CAD build for the part. Positions are in the model's coordinates, mm. Face numbers are marked on the shaded views. A direction names the side the tool comes from. Give positions to 0.01 mm unless a question says otherwise; leave off trailing zeros. Write each loop counter-clockwise with the first axis right and the second up, starting at its lowest first coordinate (ties: lowest second). Pieces come first, ordered by that corner, then holes. Notation, with made-up numbers: M -12,-25 L 22,-25 A30 ccw 22,14 Z; hole C 54.25,79.5 d7. An arc over 180 degrees is marked long. One line per question, with ' | ' between items. Start each with the question number.
1. Cut at A-A, the plane z = 0. Write the cut outline in (x, y).
2. Cut at B-B, the plane y = 10.5. Write the cut outline in (x, z).
3. Cut at D-D, the plane y = 5.75. Write the cut outline in (x, z), then the cut area to 3 significant figures.
4. Which spindle directions (+Z, -Z, +X, -X, +Y, -Y) get a long thin tool onto all of the face, cutting with end or side? Do the marked faces 1 and 2. Say none if no direction does.
5. Flat gauge pins, fed straight in: pin 1 (8 mm diameter, centred on x = 29.5, z = 37.5, fed in from +Y); pin 2 (5 mm diameter, centred on x = 10.5, y = 6, fed in from -Z); pin 3 (0.6 mm diameter, centred on y = 3, z = 0, fed in from +X); pin 4 (3.5 mm diameter, centred on x = 0, z = 0, fed in from +Y). Where does each tip first touch, or does it go through?
6. Wall check: L1, parallel to X at y = 3.2, z = 0; L2, parallel to X at y = 1.5, z = 0; L3, parallel to Z at x = -1, y = 3. Give the ranges that are in metal, low to high.
7. Cut at C-C, the plane x = 0. Write the cut outline in (y, z), then the cut area to 3 significant figures.
```python
from build123d import *

# Parameters (mm, degrees)
BOSS_EXTRUDE1_DEPTH = 9
SKETCH2_W           = 4
SKETCH2_H           = 20
BOSS_EXTRUDE2_DEPTH = 17
SKETCH3_W           = 15
SKETCH3_H           = 5
CUT_EXTRUDE1_DEPTH  = 66.094162565
SKETCH4_R           = 3
CUT_EXTRUDE2_DEPTH  = 68.830671528
CUT_EXTRUDE3_DEPTH  = 73.919476136
CUT_EXTRUDE4_DEPTH  = 71.606302835
FILLET1_R           = 5
CHAMFER1_SIZE       = 2


with BuildPart() as part:
    # Sketch1 → Boss-Extrude1 (new body)
    with BuildSketch(Plane(origin=(0, 0, 0), x_dir=(1, 0, 0), z_dir=(0, 1, 0))):
        Polygon((7.5, -7.5), (36, -36), (36, -51), (-7.5, -7.5), (-7.5, 7.5), (7.5, 7.5), align=None)
    extrude(amount=BOSS_EXTRUDE1_DEPTH)

    # Sketch2 → Boss-Extrude2 (add)
    with BuildSketch(Plane.XZ):
        with Locations((34, 46)):
            Rectangle(SKETCH2_W, SKETCH2_H)
    extrude(amount=-BOSS_EXTRUDE2_DEPTH)

    # Sketch3 → Cut-Extrude1 (cut, through all)
    with BuildSketch(Plane(origin=(7.5, 0, 0), x_dir=(0, 0, -1), z_dir=(1, 0, 0))):
        with Locations((0, 6.5)):
            Rectangle(SKETCH3_W, SKETCH3_H)
    extrude(amount=-CUT_EXTRUDE1_DEPTH, mode=Mode.SUBTRACT)

    # Sketch4 → Cut-Extrude2 (cut, through all)
    with BuildSketch(Plane(origin=(0, 4, 0), x_dir=(1, 0, 0), z_dir=(0, 1, 0))):
        with Locations(Location((0, 0, 0), (0, 0, 270))):
            Circle(SKETCH4_R)
    extrude(amount=-CUT_EXTRUDE2_DEPTH, mode=Mode.SUBTRACT)

    # Sketch5 → Cut-Extrude3 (cut, through all)
    with BuildSketch(Plane(origin=(36, 0, 0), x_dir=(0, 0, -1), z_dir=(1, 0, 0))):
        with BuildLine():
            Line((-45, 7), (-47, 7))
            ThreePointArc((-47, 7), (-50, 10), (-47, 13))
            Line((-47, 13), (-45, 13))
            ThreePointArc((-45, 13), (-42, 10), (-45, 7))
        make_face()
    extrude(amount=-CUT_EXTRUDE3_DEPTH, mode=Mode.SUBTRACT)

    # Sketch6 → Cut-Extrude4 (cut, through all)
    with BuildSketch(Plane.ZY.offset(-32)):
        with BuildLine():
            Line((47, 5), (45, 5))
            ThreePointArc((45, 5), (42.113248654, 5.917517095), (40.285954792, 8.333333333))
            ThreePointArc((40.285954792, 8.333333333), (40.917517095, 12.886751346), (45, 15))
            Line((45, 15), (47, 15))
            ThreePointArc((47, 15), (51.082482905, 12.886751346), (51.714045208, 8.333333333))
            ThreePointArc((51.714045208, 8.333333333), (49.886751346, 5.917517095), (47, 5))
        make_face()
        with BuildLine():
            Line((47, 7), (45, 7))
            ThreePointArc((45, 7), (43.267949192, 7.550510257), (42.171572875, 9))
            ThreePointArc((42.171572875, 9), (42.550510257, 11.732050808), (45, 13))
            Line((45, 13), (47, 13))
            ThreePointArc((47, 13), (49.449489743, 11.732050808), (49.828427125, 9))
            ThreePointArc((49.828427125, 9), (48.732050808, 7.550510257), (47, 7))
        make_face(mode=Mode.SUBTRACT)
    extrude(amount=CUT_EXTRUDE4_DEPTH, mode=Mode.SUBTRACT)

    # Fillet1
    fillet1_edges = [part.edges().sort_by_distance(p)[0] for p in [
        (34, 0, 56),
        (34, 17, 36),
        (34, 17, 56),
    ]]
    fillet(fillet1_edges, radius=FILLET1_R)

    # Chamfer1
    chamfer1_edges = [part.edges().sort_by_distance(p)[0] for p in [
        (21.75, 0, 21.75),
        (7.5, 0, 0),
        (0, 0, -7.5),
        (-7.5, 0, 0),
        (12.25, 0, 27.25),
        (8.800510257, 9, 23.800510257),
        (21.75, 9, 21.75),
    ]]
    chamfer(chamfer1_edges, length=CHAMFER1_SIZE)


solid = part.part
```
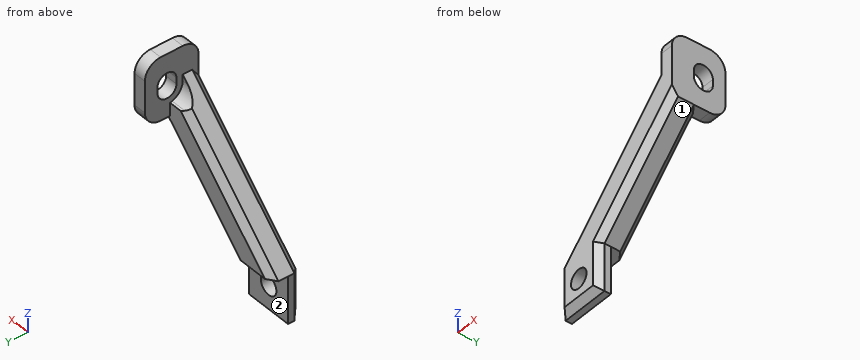
Here are the results:
1) outline: M -7.5,2 L -5.5,0 L -3,0 L -3,4 L -7.5,4 Z; M 3,0 L 5.5,0 L 7.5,2 L 7.5,4 L 3,4 Z
2) outline: M 32,36 L 36,36 L 36,42.04 L 32,42.04 Z; M 32,49.96 L 36,49.96 L 36,56 L 32,56 Z
3) outline: M -7.5,7.5 L 7.5,7.5 L 36,36 L 36,56 L 32,56 L 32,42.37 L 27.37,42.37 Z | area: 557 mm^2
4) face 1: -Z, +X, +Y, -Y | face 2: -Z, +X, -X, +Y
5) pin 1: y = 16.99 | pin 2: z = 8 | pin 3: x = 7.5 | pin 4: through
6) L1: -7.5 to -3, 3 to 7.5 | L2: -7 to -3, 3 to 7 | L3: -7.5 to -2.83, 2.83 to 14
7) outline: M 0,-5.5 L 2,-7.5 L 4,-7.5 L 4,-3 L 0,-3 Z; M 0,3 L 4,3 L 4,7.5 L 9,7.5 L 9,12.17 L 7,15 L 2,15 L 0,12.17 Z | area: 95.8 mm^2
